Autodesk Inventor part; units mm, degrees
ref_plane "YZ Plane" through (0, 0, 0) normal (1, 0, 0) x (0, 1, 0)
ref_plane "XZ Plane" through (0, 0, 0) normal (0, 1, 0) x (-1, 0, 0)
ref_plane "XY Plane" through (0, 0, 0) normal (0, 0, 1) x (1, 0, 0)
sketch "Sketch1" plane through (0, 0, 0) normal (0, 0, 1) x (1, 0, 0)
  line L0 (0, 25.4) -> (0, 0)
  line L1 (0, 0) -> (25.4, 0)
  line L2 (3.175, 25.4) -> (3.175, 4.953)
  line L3 (4.953, 3.175) -> (25.4, 3.175)
  line L4 (0, 25.4) -> (3.175, 25.4)
  line L5 (25.4, 3.175) -> (25.4, 0)
  line L6 (3.175, 4.953) -> (3.175, 3.175)
  line L7 (4.953, 3.175) -> (3.175, 3.175)
  dimension "d0" = 25.4
  dimension "d1" = 25.4
  dimension "d2" = 3.175
extrude "Extrusion1" add sketch "Sketch1" along normal blind 492.125
sketch "Sketch7" plane through (3.175, 3.175, 0) normal (1, 0, 0) x (0, 0, -1)
  circle A0 centre (-479.425, 9.525) radius 2.8124
  line L0 (0, 22.225) -> (-492.125, 22.225)
  line L1 (-492.125, 0) -> (-492.125, 22.225)
  circle A1 centre (-12.7, 9.525) radius 2.8124
  point P0 (0, -3.175)
  dimension "d43" = 12.7
  dimension "d44" = 12.7
  dimension "d47" = 466.725
hole "mount" at (3.175, 12.7, 479.425) at (3.175, 12.7, 12.7) direction (-1, 0, 0) diameter 6.7564 depth 25.4 tip angle 118
properties part number "angle_L1"
Verification items for the finished model (mm, model axes). A direction names the side the tool comes from. Give positions to 0.01 mm unless a question says otherwise; leave off trailing zeros. Order: outer loops, then holes, each group sorted by start corner. A loop starts at its lowest first (then second) coordinate and runs counter-clockwise, first axis right, second up. Notation, with made-up numbers: (-5.5, -37.5) - (42.5, -37.5) arc R23 ccw to (42.5, -0.5) - close; hole circle Ø2 at (50.25, 14.5). An arc over 180 degrees is marked (long way). Answer as CSV lines item,"result". Start each with the question number.
Item 1: Gauge pin test, flat ends, axial feed: pin 1 (4 mm diameter, centred on x = 13.5, z = 271, fed in from +Y) (3 decimals); pin 2 (6 mm diameter, centred on y = 16, z = 178.5, fed in from +X) (3 decimals). Record the tip position at first contact, or that the pin passes through.
Item 2: Section check B-B, the plane x = 11.25. Record the boundary of the cut face in (y, z) (3 decimals).
Item 3: Section check A-A, the plane z = 288. Record the boundary of the cut face in (x, y) (3 decimals).
Item 4: Access from +Z, -Z, +X, -X, +Y, -Y to the whole of each face (thin tool, end or side, straight path). Record for faces 1 (the face through (7, 2, 0)), 2 (the face through (3.175, 14, 243)).
Item 5: Material ranges on L1, parallel to Z at x = 1.2, y = 12.7 (3 decimals); L2, parallel to Y at x = 1.55, z = 12.7; L3, parallel to X at y = 3.75, z = 279.5 (3 decimals), recorded low to high.
Filled in:
1,pin 1,"y = 3.175"
1,pin 2,"x = 3.175"
2,outline,"(0, 0) - (3.175, 0) - (3.175, 492.125) - (0, 492.125) - close"
3,outline,"(0, 0) - (25.4, 0) - (25.4, 3.175) - (3.175, 3.175) - (3.175, 25.4) - (0, 25.4) - close"
4,face 1,"-Z, +X, -X, +Y, -Y"
4,face 2,"+Z, -Z, +X, +Y"
5,L1,"0 to 9.322, 16.078 to 476.047, 482.803 to 492.125"
5,L2,"0 to 9.32, 16.08 to 25.4"
5,L3,"0 to 3.175"
